For this review, use the dimensioned drawing (mm, ordinates from the lowest corner) and the shaded views. Give positions to 0.01 mm unless a question says otherwise; leave off trailing zeros. Write each loop counter-clockwise with the first axis right and the second up, starting at its lowest first coordinate (ties: lowest second). Pieces come first, ordered by that corner, then holes.
1) Wall thickness on line 1 along Z through (x, y) = (847, 11.5); line 2 along Z through (x, y) = (365, 1): over which ranges is each line inside the solid? List them lowest first.
2) For P1, Ø3, axis at x = 598, z = 2.5, coming from the +Y side; P2, Ø3, axis at x = 355.5, y = 11, coming from the +Z side; P3, Ø1.9, axis at x = 552.5, y = 2.5, coming from the -Z side, all flat-tipped, find the tip position at first contact; note any pin that passes through.
3) We need section A-A on x = 488.5. Give the boundary of the cut face in (y, z).
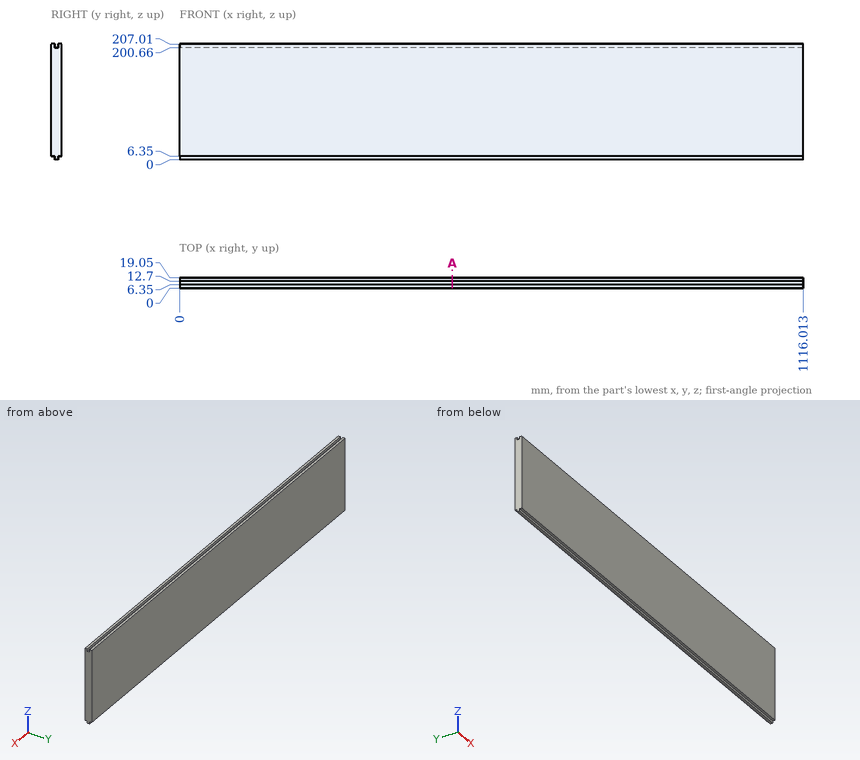
Results list:
1. line 1: z = 0 to 200.66
1. line 2: z = 6.35 to 207.01
2. P1: stops at y = 12.7
2. P2: stops at z = 200.66
2. P3: stops at z = 6.35
3. outline: (0, 6.35) - (6.35, 6.35) - (6.35, 0) - (12.7, 0) - (12.7, 6.35) - (19.05, 6.35) - (19.05, 207.01) - (12.7, 207.01) - (12.7, 200.66) - (6.35, 200.66) - (6.35, 207.01) - (0, 207.01) - close
